from build123d import *

# Parameters (mm, degrees)
EXTRUDE_THIN1_DEPTH  = 50
BOSS_EXTRUDE1_DEPTH  = 5
SKETCH5_R            = 32
SKETCH5_R_2          = 27
EXTRUDE_THIN4_DEPTH  = 17
SKETCH2_R            = 12.5
CUT_EXTRUDE2_DEPTH   = 126.505472998
BOSS_EXTRUDE4_DEPTH  = 3
FILLET1_R            = 10
FILLET2_R            = 10
BOSS_EXTRUDE5_DEPTH  = 3
FILLET3_R            = 10
FILLET4_R            = 10
BOSS_EXTRUDE11_DEPTH = 3
FILLET6_R            = 10
FILLET7_R            = 10
SKETCH14_W           = 50
SKETCH14_H           = 50
BOSS_EXTRUDE12_DEPTH = 10
CUT_EXTRUDE5_START   = -4
SKETCH16_W           = 45
SKETCH16_H           = 45
SKETCH16_R           = 13.5
SKETCH16_R_2         = 2.5
CUT_EXTRUDE5_DEPTH   = 25
SKETCH16_2_R         = 2.5
SKETCH16_2_R_2       = 13.5
CUT_EXTRUDE6_DEPTH   = 121.318842051


with BuildPart() as part:
    # Sketch1 → Extrude-Thin1 (new body)
    with BuildSketch(Plane.XY):
        with BuildLine():
            Line((-53.6900369, 50), (46.3099631, 50))
            ThreePointArc((46.3099631, 50), (96.3099631, 0), (46.3099631, -50))
            Line((46.3099631, -50), (-53.6900369, -50))
            ThreePointArc((-53.6900369, -50), (-103.6900369, 0), (-53.6900369, 50))
        make_face()
        with BuildLine():
            Line((-53.6900369, 45), (46.3099631, 45))
            ThreePointArc((46.3099631, 45), (91.3099631, 0), (46.3099631, -45))
            Line((46.3099631, -45), (-53.6900369, -45))
            ThreePointArc((-53.6900369, -45), (-98.6900369, 0), (-53.6900369, 45))
        make_face(mode=Mode.SUBTRACT)
    extrude(amount=EXTRUDE_THIN1_DEPTH)

    # Sketch1<3> → Boss-Extrude1 (add)
    with BuildSketch(Plane.XY):
        with BuildLine():
            Line((-53.6900369, -45), (46.3099631, -45))
            ThreePointArc((46.3099631, -45), (91.3099631, 0), (46.3099631, 45))
            Line((46.3099631, 45), (-53.6900369, 45))
            ThreePointArc((-53.6900369, 45), (-98.6900369, 0), (-53.6900369, -45))
        make_face()
    extrude(amount=BOSS_EXTRUDE1_DEPTH)

    # Sketch5 → Extrude-Thin4 (add)
    with BuildSketch(Plane.XY.offset(5)):
        with Locations((51.14065821, -2.257734505)):
            Circle(SKETCH5_R)
        with Locations((51.14065821, -2.257734505)):
            Circle(SKETCH5_R_2, mode=Mode.SUBTRACT)
    extrude(amount=EXTRUDE_THIN4_DEPTH)

    # Sketch2 → Cut-Extrude2 (cut, through all)
    with BuildSketch(Plane(origin=(0, 0, 0), x_dir=(-1, 0, 0), z_dir=(0, 0, -1))):
        with Locations((-51.14065821, -2.257734505)):
            Circle(SKETCH2_R)
    extrude(amount=-CUT_EXTRUDE2_DEPTH, mode=Mode.SUBTRACT)

    # Sketch10 → Boss-Extrude4 (add)
    with BuildSketch(Plane.XY.offset(5)):
        Polygon((51.14065821, 29.742265495), (46.3099631, 45), (33.078782173, 45), (40.95774875, 28.078849927), (41.321043385, 28.19838417), align=None)
    extrude(amount=BOSS_EXTRUDE4_DEPTH)

    # Fillet1
    fillet1_edges = [part.edges().sort_by_distance(p)[0] for p in [
        (40.95774875, 28.078849927, 6.5),
    ]]
    fillet(fillet1_edges, radius=FILLET1_R)

    # Fillet2
    fillet2_edges = [part.edges().sort_by_distance(p)[0] for p in [
        (51.14065821, 29.742265495, 6.5),
    ]]
    fillet(fillet2_edges, radius=FILLET2_R)

    # Sketch11 → Boss-Extrude5 (add)
    with BuildSketch(Plane.XY.offset(5)):
        Polygon((34.756480548, -29.745162946), (25.663670683, -45), (38.486673363, -45), (41.405025332, -32.740802796), align=None)
    extrude(amount=BOSS_EXTRUDE5_DEPTH)

    # Fillet3
    # the kernel refuses this fillet: 10 mm, written as the material it adds along each edge
    with BuildSketch(Plane(origin=(38.486673363, -45, 5), x_dir=(0.9995047638701084, 0.03146787252037754, 0), z_dir=(0, 0, 1))) as fillet3_piece_1:
        with BuildLine():
            CenterArc((13.052927583, 9.940340464), FILLET3_R, 167.167880579, 109.093840461)
            Line((3.302677551, 12.161291679), (2.327652547, 12.3833868))
            ThreePointArc((2.327652547, 12.3833868), (0.686292727, 6.342726217), (-0.965046048, 0.262080378))
            Line((-0.965046048, 0.262080378), (-0.031467873, -0.999504764))
            ThreePointArc((-0.031467873, -0.999504764), (7.787947488, -1.245687048), (14.252700085, -0.994034046))
            Line((14.252700085, -0.994034046), (14.143629858, 0))
        make_face()
    extrude(amount=3)

    # Fillet4
    fillet4_edges = [part.edges().sort_by_distance(p)[0] for p in [
        (25.663670683, -45, 6.5),
    ]]
    fillet(fillet4_edges, radius=FILLET4_R)

    # Sketch13 → Boss-Extrude11 (add)
    with BuildSketch(Plane.XY.offset(5)):
        Polygon((90.705735304, -8.724739526), (82.501490248, -8.724739526), (83.084727444, 0), (91.667524575, 0), align=None)
    extrude(amount=BOSS_EXTRUDE11_DEPTH)

    # Fillet6
    # the kernel refuses this fillet: 10 mm, written as the material it adds along each edge
    with BuildSketch(Plane(origin=(91.3099631, 0, 8), x_dir=(-0.13715489744354328, 0.9905496121382569, 0), z_dir=(0, 0, -1))) as fillet6_piece_1:
        with BuildLine():
            CenterArc((10.972391795, -9.905496121), FILLET6_R, 82.116754313, 87.758074962)
            Line((1.128131353, -8.147503989), (0.931246144, -8.112344146))
            ThreePointArc((0.931246144, -8.112344146), (0.365955754, -4.101182974), (-0.198109922, -0.027430979))
            Line((-0.198109922, -0.027430979), (-0.027430979, 0.198109922))
            ThreePointArc((-0.027430979, 0.198109922), (6.171970385, 0.625267454), (12.371371749, 0.198109922))
            Line((12.371371749, 0.198109922), (12.34394077, 0))
        make_face()
    extrude(amount=3)

    # Fillet7
    # the kernel refuses this fillet: 10 mm, written as the material it adds along each edge
    with BuildSketch(Plane(origin=(90.456071877, -8.724739526, 8), x_dir=(-1, 0, 0), z_dir=(0, 0, -1))) as fillet7_piece_1:
        with BuildLine():
            CenterArc((13.556604147, -8.283558638), FILLET7_R, 124.06978595, 85.005036852)
            Line((4.816745681, -13.1430724), (4.641948512, -13.240262675))
            ThreePointArc((4.641948512, -13.240262675), (1.706415001, -6.828793582), (-0.196204928, -0.03877662))
            Line((-0.196204928, -0.03877662), (0, 0.2))
            ThreePointArc((0, 0.2), (3.977290815, 0.2), (7.842541179, 0.165671173))
            Line((7.842541179, 0.165671173), (7.95458163, 0))
        make_face()
    extrude(amount=3)

    # Sketch14 → Boss-Extrude12 (add)
    with BuildSketch(Plane.XY.offset(5)):
        with Locations((-53.507483995, 0)):
            Rectangle(SKETCH14_W, SKETCH14_H)
    extrude(amount=BOSS_EXTRUDE12_DEPTH)

    # Sketch16 → Cut-Extrude5 (cut)
    with BuildSketch(Plane.XY.offset(15).offset(CUT_EXTRUDE5_START)):
        with Locations((-53.6900369, 0)):
            Rectangle(SKETCH16_W, SKETCH16_H)
        with Locations((-53.6900369, 0)):
            Circle(SKETCH16_R, mode=Mode.SUBTRACT)
        with Locations((-69.1900369, 14.04338148)):
            Circle(SKETCH16_R_2, mode=Mode.SUBTRACT)
        with Locations((-69.1900369, -16.95661852)):
            Circle(SKETCH16_R_2, mode=Mode.SUBTRACT)
        with Locations((-38.1900369, -16.95661852)):
            Circle(SKETCH16_R_2, mode=Mode.SUBTRACT)
        with Locations((-38.1900369, 14.04338148)):
            Circle(SKETCH16_R_2, mode=Mode.SUBTRACT)
    extrude(amount=-CUT_EXTRUDE5_DEPTH, mode=Mode.SUBTRACT)

    # Sketch16<2> → Cut-Extrude6 (cut, through all)
    with BuildSketch(Plane.XY.offset(15)):
        with Locations((-38.1900369, 14.04338148)):
            Circle(SKETCH16_2_R)
        with Locations((-69.1900369, 14.04338148)):
            Circle(SKETCH16_2_R)
        with Locations((-53.6900369, 0)):
            Circle(SKETCH16_2_R_2)
        with Locations((-69.1900369, -16.95661852)):
            Circle(SKETCH16_2_R)
        with Locations(Location((-38.1900369, -16.95661852, 0), (0, 0, 180))):
            Circle(SKETCH16_2_R)
    extrude(amount=-CUT_EXTRUDE6_DEPTH, mode=Mode.SUBTRACT)


solid = part.part
CAD build for the part. Positions are in the model's coordinates, mm. A direction names the side the tool comes from. Give positions to 0.01 mm unless a question says otherwise; leave off trailing zeros. Order: outer loops, then holes, each group sorted by start corner. A loop starts at its lowest first (then second) coordinate and runs counter-clockwise, first axis right, second up. Notation, with made-up numbers: (60.25, 64.5) - (116.25, 64.5) arc R7 ccw to (116.25, 71.5) - close; hole circle Ø9 at (32.5, 18.5). An arc over 180 degrees is marked (long way). Answer in a Markdown table with one row per item.
1. Flat gauge pins, fed straight in: pin 1 (1 mm diameter, centred on x = 64.5, z = 40.5, fed in from +Y); pin 2 (11 mm diameter, centred on x = 65, y = -22.5, fed in from +Z); pin 3 (6 mm diameter, centred on x = -69.19, y = -16.96, fed in from +Z); pin 4 (15 mm diameter, centred on x = -55.5, y = -4.5, fed in from +Z). Where does each tip first touch, or does it go through?
Data:
| item | result |
|---|---|
| pin 1 | stops at y = 46.77 |
| pin 2 | stops at z = 22 |
| pin 3 | stops at z = 15 |
| pin 4 | passes through |
2. Probe probe 1 along Y at (x, z) = (-17, 6); probe 2 along X at (y, z) = (25.5, 6.5); probe 3 along X at (y, z) = (41.5, 6.5). List the from-to ranges inside material, lowest first. Write a range as [from, to].
Data:
| item | result |
|---|---|
| probe 1 | y = [-50, -45], [45, 50] |
| probe 2 | x = [-96.7, -90.77], [34.78, 67.06], [83.39, 89.32] |
| probe 3 | x = [-81.58, -71.09], [34.71, 47.42], [63.71, 74.2] |
3. Pull direction Y, two halves, no side cores. Call faces 4 (the flat face through (-3, -48, 50)), 5 (the cylindrical face through (96.298, 1.099, 24.65)), 6 (the flat face through (-65, 11, 15)): pulls with the +Y half, pulls with the -Y half, needs draft (parallel to the pull), parting line crosses it, or undercut.
Data:
| item | result |
|---|---|
| face 4 | needs draft |
| face 5 | parting line crosses it |
| face 6 | undercut |
4. Saw through at D-D, the plane x = -81. Give the cut face in (y, z), plus the area to 3 significant figures.
Data:
| item | result |
|---|---|
| outline | (-41.88, 0) - (41.88, 0) - (41.88, 50) - (35.77, 50) - (35.77, 5) - (-35.77, 5) - (-35.77, 50) - (-41.88, 50) - close |
| area | 969 mm² |
5. Saw through at B-B, the plane x = -21.5. Give the cut face in (y, z).
Data:
| item | result |
|---|---|
| outline | (-50, 0) - (50, 0) - (50, 50) - (45, 50) - (45, 5) - (-45, 5) - (-45, 50) - (-50, 50) - close |
6. Tool access for faces 1 (the cylindrical face through (-66.805, 14.794, 13.028)), 2 (the flat face through (-64, 10, 11)), 3 (the cylindrical face through (37.452, 30.058, 6.521)): list every direction of +Z, -Z, +X, -X, +Y, -Y with a clear straight run to the whole face (end or side of a thin tool).
Data:
| item | result |
|---|---|
| face 1 | +Z, -Z |
| face 2 | -Z |
| face 3 | +Z |
7. Saw through at A-A, the plane z = 39. Give the cut face in (x, y), plus the area to 3 significant figures.
Data:
| item | result |
|---|---|
| outline | (-53.69, -50) - (46.31, -50) arc R50 ccw to (46.31, 50) - (-53.69, 50) arc R50 ccw to start; hole (-53.69, -45) - (46.31, -45) arc R45 ccw to (46.31, 45) - (-53.69, 45) arc R45 ccw to start |
| area | 2,490 mm² |
8. Saw through at C-C, the plane y = 5. Count the separate pieces of the cut face and the enclosed holes in it, plus the area to 3 significant figures.
Data:
| item | result |
|---|---|
| separate pieces | 3 |
| enclosed holes | 0 |
| area | 1,430 mm² |
